from build123d import *

# Parameters (mm, degrees)
ESQUISSE1_R                  = 9.25
BOSS_EXTRU_1_DEPTH           = 23.5
ESQUISSE2_R                  = 1.3
ENL_V_MAT_EXTRU_1_DEPTH      = 1
ENL_V_MAT_EXTRU_1_DEPTH_BACK = 24.5
ESQUISSE3_R                  = 4.5
ENL_V_MAT_EXTRU_2_DEPTH      = 1
ENL_V_MAT_EXTRU_2_DEPTH_BACK = 24.5
ESQUISSE4_R                  = 11.5
ESQUISSE4_R_2                = 9.25
BOSS_EXTRU_2_DEPTH           = 3
ESQUISSE5_R                  = 2.5
ENL_V_MAT_EXTRU_3_DEPTH      = 1
ENL_V_MAT_EXTRU_3_DEPTH_BACK = 24.5
BOSS_EXTRU_3_START           = -3
ESQUISSE6_R                  = 2.5
ESQUISSE6_R_2                = 1.3
BOSS_EXTRU_3_DEPTH           = 3
CONG_1_R                     = 1


with BuildPart() as part:
    # Esquisse1 → Boss.-Extru.1 (new body)
    with BuildSketch(Plane.XY):
        Circle(ESQUISSE1_R)
    extrude(amount=BOSS_EXTRU_1_DEPTH)

    # Esquisse2 → Enlèv. mat.-Extru.1 (cut, two sides)
    with BuildSketch(Plane.XY.offset(23.5)) as enl_v_mat_extru_1_sk:
        with Locations((7, 0)):
            Circle(ESQUISSE2_R)
        with Locations((0, -7)):
            Circle(ESQUISSE2_R)
        with Locations((-7, 0)):
            Circle(ESQUISSE2_R)
        with Locations((0, 7)):
            Circle(ESQUISSE2_R)
    extrude(amount=ENL_V_MAT_EXTRU_1_DEPTH, mode=Mode.SUBTRACT)
    extrude(enl_v_mat_extru_1_sk.sketch, amount=-ENL_V_MAT_EXTRU_1_DEPTH_BACK, mode=Mode.SUBTRACT)

    # Esquisse3 → Enlèv. mat.-Extru.2 (cut, two sides)
    with BuildSketch(Plane.XY.offset(23.5)) as enl_v_mat_extru_2_sk:
        Circle(ESQUISSE3_R)
    extrude(amount=ENL_V_MAT_EXTRU_2_DEPTH, mode=Mode.SUBTRACT)
    extrude(enl_v_mat_extru_2_sk.sketch, amount=-ENL_V_MAT_EXTRU_2_DEPTH_BACK, mode=Mode.SUBTRACT)

    # Esquisse4 → Boss.-Extru.2 (add)
    with BuildSketch(Plane.XY.offset(23.5)):
        Circle(ESQUISSE4_R)
        Circle(ESQUISSE4_R_2, mode=Mode.SUBTRACT)
    extrude(amount=-BOSS_EXTRU_2_DEPTH)

    # Esquisse5 → Enlèv. mat.-Extru.3 (cut, two sides)
    with BuildSketch(Plane.XY.offset(23.5)) as enl_v_mat_extru_3_sk:
        with Locations((5.656854249, 5.656854249)):
            Circle(ESQUISSE5_R)
        with Locations((5.656854249, -5.656854249)):
            Circle(ESQUISSE5_R)
        with Locations((-5.656854249, -5.656854249)):
            Circle(ESQUISSE5_R)
        with Locations((-5.656854249, 5.656854249)):
            Circle(ESQUISSE5_R)
    extrude(amount=ENL_V_MAT_EXTRU_3_DEPTH, mode=Mode.SUBTRACT)
    extrude(enl_v_mat_extru_3_sk.sketch, amount=-ENL_V_MAT_EXTRU_3_DEPTH_BACK, mode=Mode.SUBTRACT)

    # Esquisse6 → Boss.-Extru.3 (add)
    with BuildSketch(Plane.XY.offset(23.5).offset(BOSS_EXTRU_3_START)):
        with Locations((-5.656854249, 5.656854249)):
            Circle(ESQUISSE6_R)
        with Locations((-5.656854249, 5.656854249)):
            Circle(ESQUISSE6_R_2, mode=Mode.SUBTRACT)
        with Locations((5.656854249, 5.656854249)):
            Circle(ESQUISSE6_R)
        with Locations((5.656854249, 5.656854249)):
            Circle(ESQUISSE6_R_2, mode=Mode.SUBTRACT)
        with Locations((5.656854249, -5.656854249)):
            Circle(ESQUISSE6_R)
        with Locations((5.656854249, -5.656854249)):
            Circle(ESQUISSE6_R_2, mode=Mode.SUBTRACT)
        with Locations((-5.656854249, -5.656854249)):
            Circle(ESQUISSE6_R)
        with Locations((-5.656854249, -5.656854249)):
            Circle(ESQUISSE6_R_2, mode=Mode.SUBTRACT)
    extrude(amount=BOSS_EXTRU_3_DEPTH)

    # Congé1
    cong_1_edges = [part.edges().sort_by_distance(p)[0] for p in [
        (7.966686716, 4.700468356, 10.25),
        (4.700468356, 7.966686716, 10.25),
        (4.700468356, -7.966686716, 10.25),
        (7.966686716, -4.700468356, 10.25),
        (-7.966686716, -4.700468356, 10.25),
        (-4.700468356, -7.966686716, 10.25),
        (-4.700468356, 7.966686716, 10.25),
        (-7.966686716, 4.700468356, 10.25),
    ]]
    fillet(cong_1_edges, radius=CONG_1_R)


solid = part.part
For this review, take the finished solid that the model builds, in its own axes (mm). A direction names the side the tool comes from. Round coordinates to 2 decimals unless told otherwise and drop trailing zeros. Loops run counter-clockwise (first coordinate to the right, second up) from the corner with the lowest first, then second, coordinate; pieces in that order, holes last. Notation, with made-up numbers: (-18, -22.75) - (38, -22.75) arc R24 ccw to (38, -10.75) - close; hole circle Ø10 at (83.25, 28). An arc over 180 degrees is marked (long way). Put each result on its own line as item: value. Start each with the question number.
1. For faces 1 (the cylindrical face through (0.05, 9.25, 10.11)), 2 (the cylindrical face through (-3.854, -3.925, 10.394)), 3 (the cylindrical face through (-5.94, 4.39, 21.98)), 4 (the cylindrical face through (-0.05, -9.25, 10.11)), 5 (the cylindrical face through (-9.25, 0.05, 10.11)), list the 3-axis set-ups (+Z, -Z, +X, -X, +Y, -Y) from which the entire face can be reached by the end or side of a thin tool; tool diameter is ignored.
2. Consider section C-C on y = -5. State the section outline as (x, z) points (3 decimals).
3. For probe 1 along X at (y, z) = (1, 21); probe 2 along Z at (x, y) = (-5.5, -8); probe 3 along X at (y, z) = (6.25, 8), list the stretches that pass through material, from the lowest coordinate up. Write a range as [from, to].
4. Insertion check: P1, Ø8, axis at x = -8, z = 4.5, coming from the -Y side; P2, Ø1.6, axis at x = 5.66, y = 5.66, coming from the -Z side; P3, Ø4, axis at x = -5.66, y = 5.66, coming from the -Z side; P4, Ø1.5, axis at x = 2, z = 20.5, coming from the +Y side. Each pin has a flat end and moves straight along its axis. Give the tip position at first contact, or say it passes through.
5. Consider section A-A on y = 0. State the section outline as (x, z) points, plus the area to 3 significant figures.
6. Consider section D-D on z = 21.25. State how many separate pieces and enclosed holes the cut face has, plus the area to 3 significant figures.
7. Mouldability with a two-part tool opening along X and no side actions: class faces 6 (the cylindrical face through (8.24, 0.39, 11.91)), 7 (the flat face through (-4.2, -2, 0)), 8 (the cylindrical face through (9.25, -0.05, 10.11)) as +X half, -X half, draft (parallel to the pull), parting line (faces both ways), or undercut.
Result sheet:
1. face 1: -Z, +Y
1. face 2: -Z
1. face 3: +Z, -Z
1. face 4: -Z, -Y
1. face 5: -Z, -X
2. outline: (-10.356, 20.5) - (-6.779, 20.5) - (-6.779, 23.5) - (-10.356, 23.5) - close; (-4.535, 20.5) - (-3.245, 20.5) - (-3.245, 0) - (3.245, 0) - (3.245, 20.5) - (4.535, 20.5) - (4.535, 23.5) - (-4.535, 23.5) - close; (6.779, 20.5) - (10.356, 20.5) - (10.356, 23.5) - (6.779, 23.5) - close
3. probe 1: [-11.46, -7.83], [-6.17, -4.39], [4.39, 6.17], [7.83, 11.46]
3. probe 2: [20.5, 23.5]
3. probe 3: [-3.23, -1.06], [1.06, 3.23]
4. P1: y = -3.85
4. P2: through
4. P3: z = 20.5
4. P4: y = 11.43
5. outline: (-11.5, 20.5) - (-9.25, 20.5) - (-9.25, 0) - (-8.3, 0) - (-8.3, 23.5) - (-11.5, 23.5) - close; (-5.7, 0) - (-4.5, 0) - (-4.5, 23.5) - (-5.7, 23.5) - close; (4.5, 0) - (5.7, 0) - (5.7, 23.5) - (4.5, 23.5) - close; (8.3, 0) - (9.25, 0) - (9.25, 20.5) - (11.5, 20.5) - (11.5, 23.5) - (8.3, 23.5) - close
5. area: 115 mm^2
6. separate pieces: 1
6. enclosed holes: 9
6. area: 309 mm^2
7. face 6: undercut
7. face 7: draft
7. face 8: +X half
